```python
from build123d import *

# Parameters (mm, degrees)
CROQUIS1_W                 = 80.6
CROQUIS1_H                 = 36
CROQUIS1_R                 = 1.5
SALIENTE_EXTRUIR1_DEPTH    = 2
CROQUIS2_W                 = 71
CROQUIS2_H                 = 24.5
SALIENTE_EXTRUIR2_DEPTH    = 7
CROQUIS3_W                 = 63.6
CROQUIS3_H                 = 15
CORTAR_EXTRUIR1_DEPTH      = 0.5
CORTAR_EXTRUIR2_DEPTH      = 30.5
CORTAR_EXTRUIR2_DEPTH_BACK = 30.5
SALIENTE_EXTRUIR3_DEPTH    = 3.5
CROQUIS6_R                 = 0.5
CORTAR_EXTRUIR3_DEPTH      = 3.5
CROQUIS8_R                 = 0.5
CORTAR_EXTRUIR4_DEPTH      = 0.05
MATRIZL1_COUNT             = 16
MATRIZL1_PITCH             = 2.5


with BuildPart() as part:
    # Croquis1 → Saliente-Extruir1 (new body)
    with BuildSketch(Plane.XY):
        Rectangle(CROQUIS1_W, CROQUIS1_H)
        with Locations((37.8, 15.5)):
            Circle(CROQUIS1_R, mode=Mode.SUBTRACT)
        with Locations((-37.8, 15.5)):
            Circle(CROQUIS1_R, mode=Mode.SUBTRACT)
        with Locations((37.8, -15.5)):
            Circle(CROQUIS1_R, mode=Mode.SUBTRACT)
        with Locations((-37.8, -15.5)):
            Circle(CROQUIS1_R, mode=Mode.SUBTRACT)
    extrude(amount=SALIENTE_EXTRUIR1_DEPTH)

    # Croquis2 → Saliente-Extruir2 (add)
    with BuildSketch(Plane.XY.offset(2)):
        with Locations((0.2, -0.25)):
            Rectangle(CROQUIS2_W, CROQUIS2_H)
    extrude(amount=SALIENTE_EXTRUIR2_DEPTH)

    # Croquis3 → Cortar-Extruir1 (cut)
    with BuildSketch(Plane.XY.offset(9)):
        Rectangle(CROQUIS3_W, CROQUIS3_H)
    extrude(amount=-CORTAR_EXTRUIR1_DEPTH, mode=Mode.SUBTRACT)

    # Croquis4 → Cortar-Extruir2 (cut, two sides)
    with BuildSketch(Plane(origin=(0, 0, 0), x_dir=(0, 0, -1), z_dir=(1, 0, 0))) as cortar_extruir2_sk:
        with BuildLine():
            Line((-9, 10.401372799), (-9, 9.098123873))
            ThreePointArc((-9, 9.098123873), (-8.348627201, 9.75), (-9, 10.401372799))
        make_face()
        with BuildLine():
            ThreePointArc((-9, -9.098627201), (-8.348627201, -9.75), (-9, -10.401372799))
            Line((-9, -10.401372799), (-9, -9.098627201))
        make_face()
    extrude(amount=CORTAR_EXTRUIR2_DEPTH, mode=Mode.SUBTRACT)
    extrude(cortar_extruir2_sk.sketch, amount=-CORTAR_EXTRUIR2_DEPTH_BACK, mode=Mode.SUBTRACT)

    # Croquis5 → Saliente-Extruir3 (add)
    with BuildSketch(Plane.XY.offset(2)):
        Polygon((35.7, 4.25), (40.3, 2.25), (40.3, -2.75), (35.7, -4.75), align=None)
    extrude(amount=SALIENTE_EXTRUIR3_DEPTH)

    # Croquis6 → Cortar-Extruir3 (cut)
    with BuildSketch(Plane.XY.offset(2)):
        with Locations((-32.3, 15)):
            Circle(CROQUIS6_R)
        with Locations((-29.8, 15)):
            Circle(CROQUIS6_R)
        with Locations((-27.3, 15)):
            Circle(CROQUIS6_R)
        with Locations((-24.8, 15)):
            Circle(CROQUIS6_R)
        with Locations((-22.3, 15)):
            Circle(CROQUIS6_R)
        with Locations((-19.8, 15)):
            Circle(CROQUIS6_R)
        with Locations((-17.3, 15)):
            Circle(CROQUIS6_R)
        with Locations((-14.8, 15)):
            Circle(CROQUIS6_R)
        with Locations((-12.3, 15)):
            Circle(CROQUIS6_R)
        with Locations((-9.8, 15)):
            Circle(CROQUIS6_R)
        with Locations((-7.3, 15)):
            Circle(CROQUIS6_R)
        with Locations((-4.8, 15)):
            Circle(CROQUIS6_R)
        with Locations((-2.3, 15)):
            Circle(CROQUIS6_R)
        with Locations((0.2, 15)):
            Circle(CROQUIS6_R)
        with Locations((2.7, 15)):
            Circle(CROQUIS6_R)
        with Locations((5.2, 15)):
            Circle(CROQUIS6_R)
    extrude(amount=-CORTAR_EXTRUIR3_DEPTH, mode=Mode.SUBTRACT)

    # Croquis8 → Cortar-Extruir4 (cut)
    with BuildSketch(Plane.XY.offset(2)):
        with BuildLine():
            Line((-33.2, 15), (-33.2, 18))
            Line((-33.2, 18), (-31.4, 18))
            Line((-31.4, 18), (-31.4, 15))
            ThreePointArc((-31.4, 15), (-32.3, 14.1), (-33.2, 15))
        make_face()
        with Locations((-32.3, 15)):
            Circle(CROQUIS8_R, mode=Mode.SUBTRACT)
    cortar_extruir4 = extrude(amount=-CORTAR_EXTRUIR4_DEPTH, mode=Mode.SUBTRACT)

    # MatrizL1: Cortar-Extruir4 ×16
    with Locations(*[(i * MATRIZL1_PITCH, 0, 0) for i in range(1, MATRIZL1_COUNT)]):
        add(cortar_extruir4, mode=Mode.SUBTRACT)


solid = part.part
```
Work out the finished part from the listing and answer in its coordinate system (mm). A direction names the side the tool comes from. Round coordinates to 2 decimals unless told otherwise and drop trailing zeros. Write each loop counter-clockwise with the first axis right and the second up, starting at its lowest first coordinate (ties: lowest second). Pieces come first, ordered by that corner, then holes. Notation, with made-up numbers: (-40, 82.25) - (-5, 82.25) arc R12 cw to (-5, 87.25) - close; hole circle Ø1 at (-3.5, 47.25). An arc over 180 degrees is marked (long way). Return JSON: item names as keys, results as strings. Group by question number.
Q1. The mould has two halves that part along Y. Classify faces 1 (the cylindrical face through (39.23, 15.95, 0.99)), 2 (the flat face through (-15, 16, 1.95)), 3 (the flat face through (-1, 18, 1)): released by +Y, released by -Y, zero draft, split by the parting line, or undercut.
Q2. The part is cut by section C-C on x = 37.8. Write down the section's boundary in (y, z).
Q3. Each of these flat-tipped pins is pushed along its axis until it touches: pin 1 Ø3.5 at (y, z) = (3.5, 5) entering from -X; pin 2 Ø5 at (x, z) = (23.5, 5) entering from -Y; pin 3 Ø2 at (x, y) = (-17, -2.5) entering from +Z. Where does it stop, or does it pass through?
Q4. The part is cut by section D-D on z = 6.5. Write down the section's boundary in (x, y).
Q5. For faces 4 (the flat face through (0, 0, 8.5)), 5 (the flat face through (-35.3, 0, 5)), 6 (the flat face through (0, -12.5, 5)), determine the directions among +Z, -Z, +X, -X, +Y, -Y from which every point of the face is accessible in a straight line to the end or side of a thin tool.
Q6. The part is cut by section A-A on x = 16. Write down the section's boundary in (y, z).
Q7. Find the intervals of material crossed by L1, parallel to Y at x = -37.8, z = 1.2; L2, parallel to Y at x = -24.8, z = 0.95; L3, parallel to Z at x = -18.5, y = -3, in increasing order.
Q8. The part is cut by section B-B on y = -11.5. Write down the section's boundary in (x, z), then the cut area to 3 significant figures.
Solved:
{
 "1": {"face 1": "undercut", "face 2": "zero draft", "face 3": "released by +Y"},
 "2": {"outline": "(-18, 0) - (-17, 0) - (-17, 2) - (-18, 2) - close; (-14, 0) - (14, 0) - (14, 2) - (3.34, 2) - (3.34, 5.5) - (-3.84, 5.5) - (-3.84, 2) - (-14, 2) - close; (17, 0) - (18, 0) - (18, 2) - (17, 2) - close"},
 "3": {"pin 1": "x = -35.3", "pin 2": "y = -12.5", "pin 3": "z = 8.5"},
 "4": {"outline": "(-35.3, -12.5) - (35.7, -12.5) - (35.7, 12) - (-35.3, 12) - close"},
 "5": {"face 4": "+Z", "face 5": "+Z, -X, +Y, -Y", "face 6": "+Z, +X, -X, -Y"},
 "6": {"outline": "(-18, 0) - (18, 0) - (18, 2) - (12, 2) - (12, 9) - (10.4, 9) arc R0.65 cw to (9.1, 9) - (7.5, 9) - (7.5, 8.5) - (-7.5, 8.5) - (-7.5, 9) - (-9.1, 9) arc R0.65 cw to (-10.4, 9) - (-12.5, 9) - (-12.5, 2) - (-18, 2) - close"},
 "7": {"L1": "-18 to -17, -14 to 14, 17 to 18", "L2": "-18 to 14.5, 15.5 to 18", "L3": "0 to 8.5"},
 "8": {"outline": "(-40.3, 0) - (40.3, 0) - (40.3, 2) - (35.7, 2) - (35.7, 9) - (-35.3, 9) - (-35.3, 2) - (-40.3, 2) - close", "area": "658 mm²"}
}
